from build123d import *

# Parameters (mm, degrees)
LINK_EYE_SHELF_START          = -14.5
SKETCH1_W                     = 12
SKETCH1_H                     = 9
SKETCH1_R                     = 1.05
LINK_EYE_SHELF_DEPTH          = 2
OUTBOARD_WEB_START            = -13.5
SKETCH2_W                     = 12
SKETCH2_H                     = 3
OUTBOARD_WEB_DEPTH            = 12.5
INTERMEDIATE_PLATE_FOOT_START = -2
SKETCH3_W                     = 12
SKETCH3_H                     = 10
SKETCH3_R                     = 1.45
INTERMEDIATE_PLATE_FOOT_DEPTH = 2
CHAMFER1_SIZE                 = 1.15


with BuildPart() as part:
    # Sketch1 → Link_Eye_Shelf (new body)
    with BuildSketch(Plane.XY.offset(LINK_EYE_SHELF_START)):
        with Locations((-20, 35.5)):
            Rectangle(SKETCH1_W, SKETCH1_H)
        with Locations((-20, 36)):
            Circle(SKETCH1_R, mode=Mode.SUBTRACT)
    extrude(amount=LINK_EYE_SHELF_DEPTH)

    # Sketch2 → Outboard_Web (add)
    with BuildSketch(Plane.XY.offset(OUTBOARD_WEB_START)):
        with Locations((-20, 32.5)):
            Rectangle(SKETCH2_W, SKETCH2_H)
    extrude(amount=OUTBOARD_WEB_DEPTH)

    # Sketch3 → Intermediate_Plate_Foot (add)
    with BuildSketch(Plane.XY.offset(INTERMEDIATE_PLATE_FOOT_START)):
        with Locations((-20, 29)):
            Rectangle(SKETCH3_W, SKETCH3_H)
        with Locations((-23, 27)):
            Circle(SKETCH3_R, mode=Mode.SUBTRACT)
        with Locations((-17, 27)):
            Circle(SKETCH3_R, mode=Mode.SUBTRACT)
    extrude(amount=INTERMEDIATE_PLATE_FOOT_DEPTH)

    # Chamfer1
    chamfer1_edges = [part.edges().sort_by_distance(p)[0] for p in [
        (-18.45, 27, -2),
        (-24.45, 27, -2),
    ]]
    chamfer(chamfer1_edges, length=CHAMFER1_SIZE)


solid = part.part
Input: part model. Units: mm. Frame: model coordinates. A direction names the side the tool comes from. Coordinates: 2 decimals unless noted, no trailing zeros. Loops run counter-clockwise (first coordinate to the right, second up) from the corner with the lowest first, then second, coordinate; pieces in that order, holes last.
Q1. Cut plane C-C (x = -20). Output: boundary loops of the cut face in (y, z), then the cut area to 3 significant figures.
Q2. Draft query along X for faces 1 (the face through (-20.1, 34.6, -14.5)), 2 (the face through (-14, 32, -7)), 3 (the face through (-22.331, 25.714, -0.431)). Return one class per face: +X half, -X half, draft (parallel to the pull), parting line (faces both ways), or undercut.
Q3. Cut plane D-D (z = -11). Output: boundary loops of the cut face in (x, y), then the cut area to 3 significant figures.
Q4. Cut plane A-A (x = -23). Output: boundary loops of the cut face in (y, z), then the cut area to 3 significant figures.
Q5. Cut plane B-B (y = 27). Output: boundary loops of the cut face in (x, z).
Q6. Set-up query: faces 4 (the face through (-20, 34, -6)), 5 (the face through (-20, 31, -8)), 6 (the face through (-20, 29, 0)). Return all of +Z, -Z, +X, -X, +Y, -Y with unobstructed straight access to the full face (end or side cutting, diameter ignored); none if empty.
Q7. Contact query for flat-ended pins moving along their axis: pin 1 (4 mm diameter, centred on x = -23, z = -7.5, fed in from -Y); pin 2 (1 mm diameter, centred on x = -17.5, z = -5, fed in from +Y); pin 3 (2.5 mm diameter, centred on x = -20, y = 36, fed in from +Z). Output: stop coordinate, or through.
Q8. Material intervals for line 1 (Y direction, x = -17, z = -0.35); line 2 (Y direction, x = -20, z = -13); line 3 (Z direction, x = -20.75, y = 25.25), sorted ascending.
Working result:
1. outline: (24, -2) - (31, -2) - (31, -14.5) - (34.95, -14.5) - (34.95, -12.5) - (34, -12.5) - (34, 0) - (24, 0) - close; (37.05, -14.5) - (40, -14.5) - (40, -12.5) - (37.05, -12.5) - close
1. area: 65.3 mm2
2. face 1: draft
2. face 2: +X half
2. face 3: undercut
3. outline: (-26, 31) - (-14, 31) - (-14, 34) - (-26, 34) - close
3. area: 36.0 mm2
4. outline: (24, -2) - (24.4, -2) - (25.55, -0.85) - (25.55, 0) - (24, 0) - close; (28.45, -0.85) - (29.6, -2) - (31, -2) - (31, -14.5) - (40, -14.5) - (40, -12.5) - (34, -12.5) - (34, 0) - (28.45, 0) - close
4. area: 62.4 mm2
5. outline: (-26, -2) - (-25.6, -2) - (-24.45, -0.85) - (-24.45, 0) - (-26, 0) - close; (-21.55, -0.85) - (-20.4, -2) - (-19.6, -2) - (-18.45, -0.85) - (-18.45, 0) - (-21.55, 0) - close; (-15.55, -0.85) - (-14.4, -2) - (-14, -2) - (-14, 0) - (-15.55, 0) - close
6. face 4: +Z, +X, -X, +Y
6. face 5: -Z, +X, -X, -Y
6. face 6: +Z, +X, -X, +Y, -Y
7. pin 1: stops at y = 31
7. pin 2: stops at y = 34
7. pin 3: stops at z = -12.5
8. line 1: y = 24 to 25.55, 28.45 to 34
8. line 2: y = 31 to 34.95, 37.05 to 40
8. line 3: z = -2 to 0
